```python
from build123d import *

# Parameters (mm, degrees)
SKETCH1_W           = 50
SKETCH1_H           = 35
SKETCH1_R           = 11
SKETCH1_R_2         = 3
BOSS_EXTRUDE1_DEPTH = 5
SKETCH2_W           = 32
SKETCH2_H           = 30
SKETCH2_H_2         = 5
BOSS_EXTRUDE2_DEPTH = 3
SKETCH3_W           = 35
SKETCH3_H           = 38
BOSS_EXTRUDE3_DEPTH = 2
FILLET1_R           = 5


with BuildPart() as part:
    # Sketch1 → Boss-Extrude1 (new body)
    with BuildSketch(Plane.XY):
        Rectangle(SKETCH1_W, SKETCH1_H)
        with Locations((-9, 0)):
            Circle(SKETCH1_R, mode=Mode.SUBTRACT)
        with Locations(Location((16, -10, 0), (0, 0, 180))):
            Circle(SKETCH1_R_2, mode=Mode.SUBTRACT)
        with Locations((16, 10)):
            Circle(SKETCH1_R_2, mode=Mode.SUBTRACT)
    extrude(amount=BOSS_EXTRUDE1_DEPTH)

    # Sketch2 → Boss-Extrude2 (add)
    with BuildSketch(Plane(origin=(0, 17.5, 0), x_dir=(1, 0, 0), z_dir=(0, 1, 0))):
        with Locations((-9, 15)):
            Rectangle(SKETCH2_W, SKETCH2_H)
        with Locations((-9, -2.5)):
            Rectangle(SKETCH2_W, SKETCH2_H_2)
    extrude(amount=BOSS_EXTRUDE2_DEPTH)

    # Sketch3 → Boss-Extrude3 (add)
    with BuildSketch(Plane.ZY.offset(25)):
        with Locations((-12.5, 1.5)):
            Rectangle(SKETCH3_W, SKETCH3_H)
    extrude(amount=BOSS_EXTRUDE3_DEPTH)

    # Fillet1
    # the kernel refuses this fillet: 5 mm, written as the material it adds along each edge
    with BuildSketch(Plane(origin=(7, 17.5, 5), x_dir=(1, 0, 0), z_dir=(0, 0, -1))) as fillet1_piece_1:
        with BuildLine():
            CenterArc((4.582575695, -5), FILLET1_R, 90, 66.421821522)
            Line((0, -3), (0, 0))
            Line((0, 0), (4.582575695, 0))
        make_face()
    extrude(amount=5)
    with BuildSketch(Plane(origin=(-25, 17.5, -30), x_dir=(0, -1, 0), z_dir=(0, 0, 1))) as fillet1_piece_2:
        with BuildLine():
            CenterArc((FILLET1_R, FILLET1_R), FILLET1_R, 180, 90)
            Line((0, FILLET1_R), (0, 0))
            Line((0, 0), (FILLET1_R, 0))
        make_face()
    extrude(amount=30)
    # the kernel refuses this fillet: 5 mm, written as the material it takes off along each edge
    with BuildSketch(Plane(origin=(25, 17.5, -12.5), x_dir=(-1, 0, 0), z_dir=(0, 0, 1)), Plane(origin=(25, -17.5, -12.5), x_dir=(0, 1, 0), z_dir=(0, 0, 1))) as fillet1_2_piece_1:
        with BuildLine():
            CenterArc((FILLET1_R, FILLET1_R), FILLET1_R, 180, 90)
            Line((0, FILLET1_R), (0, 0))
            Line((0, 0), (FILLET1_R, 0))
        make_face()
    extrude(amount=30, mode=Mode.SUBTRACT)
    with BuildSketch(Plane(origin=(-27, -17.5, -42.5), x_dir=(1, 0, 0), z_dir=(0, 0, 1))) as fillet1_2_piece_2:
        with BuildLine():
            CenterArc((FILLET1_R, FILLET1_R), FILLET1_R, 180, 90)
            Line((0, FILLET1_R), (0, 0))
            Line((0, 0), (FILLET1_R, 0))
        make_face()
    extrude(amount=60, mode=Mode.SUBTRACT)
    with BuildSketch(Plane(origin=(-27, 20.5, 17.5), x_dir=(0, -1, 0), z_dir=(0, 0, -1))) as fillet1_2_piece_3:
        with BuildLine():
            CenterArc((FILLET1_R, -FILLET1_R), FILLET1_R, 90, 90)
            Line((0, -FILLET1_R), (0, 0))
            Line((0, 0), (FILLET1_R, 0))
        make_face()
    extrude(amount=60, mode=Mode.SUBTRACT)


solid = part.part
```
Geometry: final body of the model. Coordinates: model frame, mm. A direction names the side the tool comes from. Coordinates: 2 decimals unless noted, no trailing zeros. Write each loop counter-clockwise with the first axis right and the second up, starting at its lowest first coordinate (ties: lowest second). Pieces come first, ordered by that corner, then holes. Notation, with made-up numbers: M -9.75,57 L 47.25,57 A18 cw 47.25,64 Z; hole C 22.25,17.25 d9. An arc over 180 degrees is marked long. Use CSV: the item, a comma, the result in double quotes. Start each with the question number.
1. Reachability of faces 4 (the face through (7, 19, -15)), 5 (the face through (16, 17.5, 2)), 6 (the face through (-25, -2, -15)) from +Z, -Z, +X, -X, +Y, -Y: full face, straight path, thin tool, end or side. Return the list, or none.
2. Mould query, pull axis X, two halves, no side actions, for faces 1 (the face through (-3.924, -9.759, 2.465)), 2 (the face through (23.57, 16, 2.46)), 3 (the face through (-26.554, -14.563, -12.745)). Classes: pulls with the +X half, pulls with the -X half, needs draft (parallel to the pull), parting line crosses it, or undercut.
3. Cut plane A-A on x = 16. Return the cut outline in (y, z), plus the area to 3 significant figures.
4. Ray query, probe 1 along Y at (x, z) = (16, 1); probe 2 along X at (y, z) = (-10, 3.9); probe 3 along Y at (x, z) = (-16, -3). Return the intervals inside material, ascending.
5. First-contact query: P1, Ø8, axis at x = 16, y = -10, coming from the +Z side; P2, Ø14.5, axis at y = 1.5, z = -21.5, coming from the +X side; P3, Ø4, axis at x = -12.5, z = -17, coming from the -Y side; P4, Ø2.5, axis at x = 16, z = 1.5, coming from the +Y side. Flat tips, straight axial feed; report the tip coordinate or a pass-through.
6. Cut plane B-B on y = 0. Return the cut outline in (x, z).
7. Cut plane D-D on x = -5.5. Return the cut outline in (y, z), plus the area to 3 significant figures.
8. Cut plane C-C on z = -20.5. Return the cut outline in (x, y).
Entries:
1,face 4,"-Z, +X, +Y, -Y"
1,face 5,"+Z, -Z, +X, +Y"
1,face 6,"-Z, +X, -Y"
2,face 1,"undercut"
2,face 2,"pulls with the +X half"
2,face 3,"pulls with the -X half"
3,outline,"M -17.5,0 L -13,0 L -13,5 L -17.5,5 Z; M -7,0 L 7,0 L 7,5 L -7,5 Z; M 13,0 L 17.5,0 L 17.5,5 L 13,5 Z"
3,area,"115 mm²"
4,probe 1,"-17.5 to -13, -7 to 7, 13 to 17.5"
4,probe 2,"-27 to -13.58, -4.42 to 13, 19 to 25"
4,probe 3,"17.5 to 20.5"
5,P1,"z = 5"
5,P2,"x = -25"
5,P3,"y = 17.5"
5,P4,"y = 17.5"
6,outline,"M -27,-30 L -25,-30 L -25,0 L -20,0 L -20,5 L -27,5 Z; M 2,0 L 25,0 L 25,5 L 2,5 Z"
7,outline,"M -17.5,0 L -10.43,0 L -10.43,5 L -17.5,5 Z; M 10.43,0 L 17.5,0 L 17.5,-30 L 20.5,-30 L 20.5,5 L 10.43,5 Z"
7,area,"176 mm²"
8,outline,"M -27,-12.5 A5 ccw -25,-16.5 L -25,12.5 A5 cw -20,17.5 L 7,17.5 L 7,20.5 L -22,20.5 A5 ccw -27,15.5 Z"
